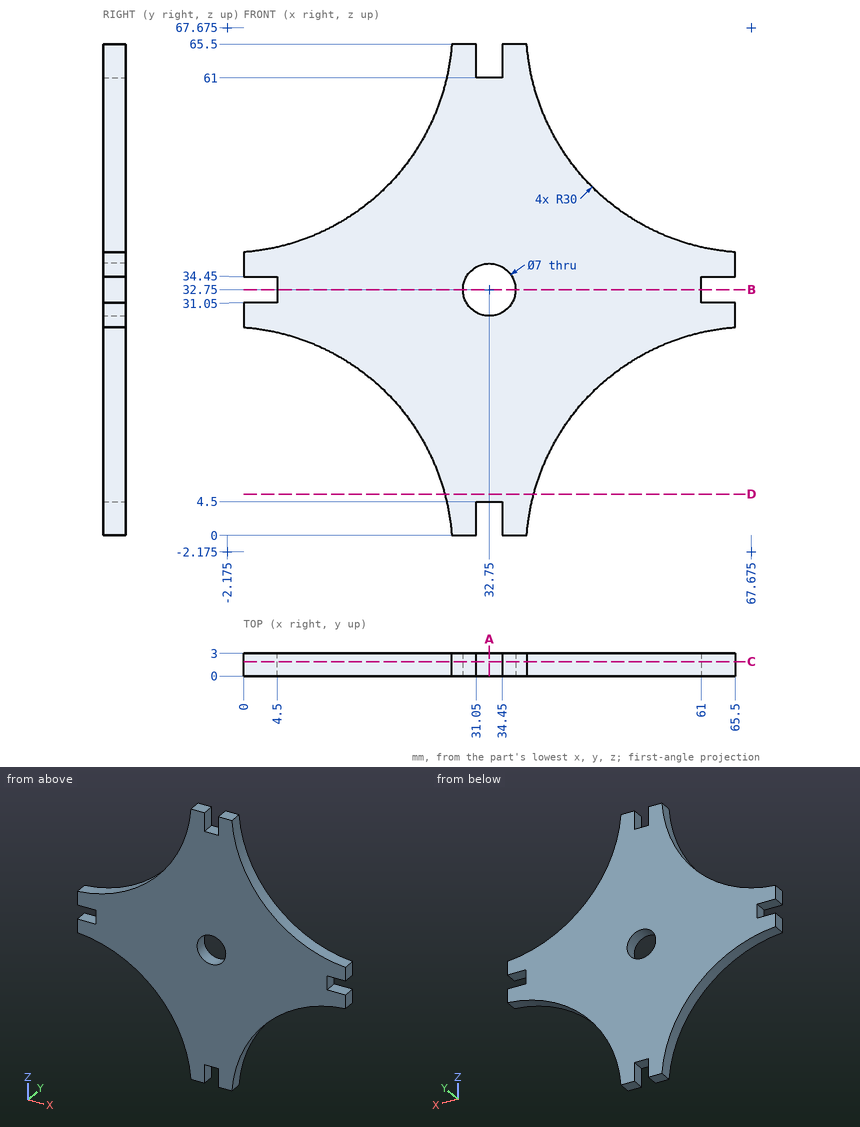
Design review of the part shown in the three views and the two pictorial views. Dimensions are in mm from the part's minimum x, y and z. Round coordinates to 2 decimals unless told otherwise and drop trailing zeros. Loops run counter-clockwise (first coordinate to the right, second up) from the corner with the lowest first, then second, coordinate; pieces in that order, holes last. Notation, with made-up numbers: (43, -32.5) - (69, -32.5) arc R14 cw to (69, -6.5) - close; hole circle Ø4 at (66, -38.5). An arc over 180 degrees is marked (long way). One line per item, written item: value. Start each with the question number.
Item 1: Take a section at A-A (x = 32.75). Give the boundary of the cut face in (y, z), plus the area to 4 significant figures.
Item 2: Take a section at C-C (y = 1.9). Give the boundary of the cut face in (x, z) (3 decimals).
Item 3: Take a section at B-B (z = 32.75). Give the boundary of the cut face in (x, y), plus the area to 4 significant figures.
Item 4: For L1, parallel to X at y = 0.7, z = 32.75; L2, parallel to X at y = 0.65, z = 62, list the stretches that pass through material, from the lowest coordinate up.
Item 5: Take a section at D-D (z = 5.5). Give the boundary of the cut face in (x, y), plus the area to 3 significant figures.
Item 6: Clearance check with flat-ended pins moving along their axes: pin 1 Ø0.9 at (x, y) = (64.5, 1.5) entering from +Z; pin 2 Ø1 at (y, z) = (1.5, 9.5) entering from -X; pin 3 Ø0.9 at (y, z) = (2, 2.5) entering from -X; pin 4 Ø4 at (x, z) = (32.75, 32.75) entering from +Y. State where each tip first meets the part, or that it passes through.
Answer below:
1. outline: (0, 4.5) - (3, 4.5) - (3, 29.25) - (0, 29.25) - close; (0, 36.25) - (3, 36.25) - (3, 61) - (0, 61) - close
1. area: 148.5 mm2
2. outline: (0, 27.746) arc R30 cw to (27.746, 0) - (31.05, 0) - (31.05, 4.5) - (34.45, 4.5) - (34.45, 0) - (37.754, 0) arc R30 cw to (65.5, 27.746) - (65.5, 31.05) - (61, 31.05) - (61, 34.45) - (65.5, 34.45) - (65.5, 37.754) arc R30 cw to (37.754, 65.5) - (34.45, 65.5) - (34.45, 61) - (31.05, 61) - (31.05, 65.5) - (27.746, 65.5) arc R30 cw to (0, 37.754) - (0, 34.45) - (4.5, 34.45) - (4.5, 31.05) - (0, 31.05) - close; hole circle Ø7 at (32.75, 32.75)
3. outline: (4.5, 0) - (29.25, 0) - (29.25, 3) - (4.5, 3) - close; (36.25, 0) - (61, 0) - (61, 3) - (36.25, 3) - close
3. area: 148.5 mm2
4. L1: x = 4.5 to 29.25, 36.25 to 61
4. L2: x = 27.28 to 31.05, 34.45 to 38.22
5. outline: (26.83, 0) - (38.67, 0) - (38.67, 3) - (26.83, 3) - close
5. area: 35.5 mm2
6. pin 1: stops at z = 37.89
6. pin 2: stops at x = 25.24
6. pin 3: stops at x = 27.38
6. pin 4: passes through
